Here's how the part is built. I have some questions about the finished solid (model axes, mm). Face numbers are marked on the shaded views. A direction names the side the tool comes from. Round coordinates to 2 decimals unless told otherwise and drop trailing zeros. Loops run counter-clockwise (first coordinate to the right, second up) from the corner with the lowest first, then second, coordinate; pieces in that order, holes last. Notation, with made-up numbers: M 87.25,23.25 L 96.25,23.25 A31 ccw 96.25,58.25 Z; hole C 67,23.5 d11. An arc over 180 degrees is marked long. Answer as a JSON object with one key per item and string values.
from build123d import *

# Parameters (mm, degrees)
BOSS_EXTRUDE1_DEPTH = 7.5
BOSS_EXTRUDE2_DEPTH = 7.5
DRAFT2_START        = -54.946043165
DRAFT2_DEPTH        = 100
DRAFT2_2_DEPTH      = 25
DRAFT2_START_2      = -29.946043165
DRAFT2_3_DEPTH      = 25
DRAFT2_START_3      = -4.946043165
DRAFT2_4_DEPTH      = 25
DRAFT2_START_4      = 20.053956835
DRAFT2_5_DEPTH      = 25
DRAFT2_START_5      = 35.053956835
DRAFT2_6_DEPTH      = 30
DRAFT2_START_6      = 65.053956835
DRAFT2_7_DEPTH      = 30
SKETCH3_W           = 64.747590887
SKETCH3_H           = 7.5
BOSS_EXTRUDE3_DEPTH = 7.5
CUT_EXTRUDE1_DEPTH  = 3.8
CUT_EXTRUDE2_DEPTH  = 3.8
LPATTERN1_COUNT     = 2
LPATTERN1_PITCH     = 25


# Read off the part's stored shape, not the designer's step: Draft2
with BuildPart() as part:
    # Sketch1 → Boss-Extrude1 (new body)
    with BuildSketch(Plane.XY):
        Polygon((-40.366906475, -54.946043165), (22.633093525, -54.946043165), (22.633093525, -29.946043165), (30.633093525, -29.946043165), (30.633093525, -4.946043165), (22.633093525, -4.946043165), (22.633093525, 20.053956835), (30.633093525, 20.053956835), (30.633093525, 45.053956835), (-32.366906475, 45.053956835), (-32.366906475, 20.053956835), (-40.366906475, 20.053956835), (-40.366906475, -4.946043165), (-32.366906475, -4.946043165), (-32.366906475, -29.946043165), (-40.366906475, -29.946043165), align=None)
    extrude(amount=BOSS_EXTRUDE1_DEPTH)

    # Sketch2 → Boss-Extrude2 (add)
    with BuildSketch(Plane.XY.offset(7.5)):
        Polygon((-48.166906475, 35.053956835), (30.633093525, 35.053956835), (30.633093525, 65.053956835), (38.633093525, 65.053956835), (38.633093525, 95.053956835), (-40.166906475, 95.053956835), (-40.166906475, 65.053956835), (-48.166906475, 65.053956835), align=None)
    extrude(amount=BOSS_EXTRUDE2_DEPTH)

    # Draft2 outline → Draft2 (add)
    with BuildSketch(Plane(origin=(0, 0, 0), x_dir=(1, 0, 0), z_dir=(0, 1, 0)).offset(DRAFT2_START)):
        Polygon((-32.366906475, 0), (-37.240701918, 0), (-34.803804197, -7.5), (-32.366906475, -7.5), align=None)
        Polygon((27.506888969, 0), (22.633093525, 0), (22.633093525, -7.5), (25.069991247, -7.5), align=None)
    extrude(amount=DRAFT2_DEPTH)

    # Draft2 2 outline → Draft2 2 (add)
    with BuildSketch(Plane(origin=(0, 0, 0), x_dir=(1, 0, 0), z_dir=(0, 1, 0)).offset(DRAFT2_START)):
        Polygon((-40.366906475, 0), (-45.240701918, 0), (-42.803804197, -7.5), (-40.366906475, -7.5), align=None)
    extrude(amount=DRAFT2_2_DEPTH)

    # Draft2 3 outline → Draft2 3 (add)
    with BuildSketch(Plane(origin=(0, 0, 0), x_dir=(1, 0, 0), z_dir=(0, 1, 0)).offset(DRAFT2_START_2)):
        Polygon((35.506888969, 0), (30.633093525, 0), (30.633093525, -7.5), (33.069991247, -7.5), align=None)
    extrude(amount=DRAFT2_3_DEPTH)

    # Draft2 4 outline → Draft2 4 (add)
    with BuildSketch(Plane(origin=(0, 0, 0), x_dir=(1, 0, 0), z_dir=(0, 1, 0)).offset(DRAFT2_START_3)):
        Polygon((-40.366906475, 0), (-45.240701918, 0), (-42.803804197, -7.5), (-40.366906475, -7.5), align=None)
    extrude(amount=DRAFT2_4_DEPTH)

    # Draft2 5 outline → Draft2 5 (add)
    with BuildSketch(Plane(origin=(0, 0, 0), x_dir=(1, 0, 0), z_dir=(0, 1, 0)).offset(DRAFT2_START_4)):
        Polygon((35.506888969, 0), (30.633093525, 0), (30.633093525, -7.5), (33.069991247, -7.5), align=None)
    extrude(amount=DRAFT2_5_DEPTH)

    # Draft2 6 outline → Draft2 6 (add)
    with BuildSketch(Plane(origin=(0, 0, 0), x_dir=(1, 0, 0), z_dir=(0, 1, 0)).offset(DRAFT2_START_5)):
        Polygon((-48.166906475, -15), (-48.166906475, -7.5), (-50.603804197, -7.5), align=None)
        Polygon((33.069991247, -7.5), (30.633093525, -7.5), (30.633093525, -15), align=None)
    extrude(amount=DRAFT2_6_DEPTH)

    # Draft2 7 outline → Draft2 7 (add)
    with BuildSketch(Plane(origin=(0, 0, 0), x_dir=(1, 0, 0), z_dir=(0, 1, 0)).offset(DRAFT2_START_6)):
        Polygon((41.069991247, -7.5), (38.633093525, -7.5), (38.633093525, -15), align=None)
        Polygon((-40.166906475, -7.5), (-42.603804197, -7.5), (-40.166906475, -15), align=None)
    extrude(amount=DRAFT2_7_DEPTH)

    # Sketch3 → Boss-Extrude3 (add)
    with BuildSketch(Plane(origin=(0, 0, 0), x_dir=(-1, 0, 0), z_dir=(0, 0, -1))):
        with Locations((4.866906474, -51.196043165)):
            Rectangle(SKETCH3_W, SKETCH3_H)
    boss_extrude3 = extrude(amount=BOSS_EXTRUDE3_DEPTH)

    # Sketch4 → Cut-Extrude1 (cut)
    with BuildSketch(Plane.XZ.offset(54.946043165)):
        Polygon((27.506888969, -7.5), (27.506888969, 0), (20.278859445, -2.348529157), (20.278859445, -7.5), align=None)
    cut_extrude1 = extrude(amount=-CUT_EXTRUDE1_DEPTH, mode=Mode.SUBTRACT)

    # Sketch5 → Cut-Extrude2 (cut)
    with BuildSketch(Plane(origin=(0, -47.446043165, 0), x_dir=(1, 0, 0), z_dir=(0, 1, 0))):
        Polygon((-37.240701918, 7.5), (-37.240701918, 0), (-30.012672394, 2.348529157), (-30.012672394, 7.5), align=None)
    cut_extrude2 = extrude(amount=-CUT_EXTRUDE2_DEPTH, mode=Mode.SUBTRACT)

    # LPattern1: Boss-Extrude3, Cut-Extrude1, Cut-Extrude2 ×2
    with Locations(*[(0, i * LPATTERN1_PITCH, 0) for i in range(1, LPATTERN1_COUNT)]):
        add(boss_extrude3)
        add(cut_extrude1, mode=Mode.SUBTRACT)
        add(cut_extrude2, mode=Mode.SUBTRACT)

    # Chamfer2
    # the kernel refuses this chamfer: 5 mm, written as the material it takes off along each edge
    with BuildSketch(Plane(origin=(-40.441261641, -51.612709832, 4.248239139), x_dir=(-0.7189342036162105, 0.6942471081166146, 0.033978872000742164), z_dir=(-0.4932114534551065, -0.5439749702030539, 0.6788473274406317))) as chamfer2_piece_1:
        Polygon((-3.286728939, 2.231187156), (3.915317626, 2.231187156), (-0.628588687, -4.462374312), align=None)
    extrude(amount=5.70452533, mode=Mode.SUBTRACT)
    with BuildSketch(Plane(origin=(33.069991247, -42.853897845, 7.5), x_dir=(-0.9997407638607628, 0, 0.022768510603425433), z_dir=(0, 1, 0))) as chamfer2_piece_2:
        with BuildLine():
            Line((5.163141872, 0), (-1.817393185, -4.83271311))
            Line((-1.817393185, -4.83271311), (-1.911770596, -4.799654007))
            ThreePointArc((-1.911770596, -4.799654007), (-0.947600353, -2.402729105), (-0.094377411, 0.033059103))
            Line((-0.094377411, 0.033059103), (0.002276851, 0.099974076))
            ThreePointArc((0.002276851, 0.099974076), (2.582509488, 0.041210789), (5.165418723, 0.099974076))
            Line((5.165418723, 0.099974076), (5.163141872, 0))
        make_face()
    extrude(amount=50.815709359, mode=Mode.SUBTRACT)
    with BuildSketch(Plane(origin=(-49.214170654, -54.946043165, -12.229079318), x_dir=(0.9506969379377622, -0.027495876610586285, -0.30890016018962835), z_dir=(0.309016994289291, 0, 0.951056516322985))) as chamfer2_piece_3:
        with BuildLine():
            Line((5.143365976, 0), (-0.282735774, 5.135588968))
            Line((-0.282735774, 5.135588968), (-0.382697966, 5.13283938))
            ThreePointArc((-0.382697966, 5.13283938), (-0.170646135, 2.566989148), (-0.099962192, -0.002749588))
            Line((-0.099962192, -0.002749588), (0.002749588, -0.099962192))
            ThreePointArc((0.002749588, -0.099962192), (2.572488324, -0.029278248), (5.146115564, -0.099962192))
            Line((5.146115564, -0.099962192), (5.143365976, 0))
        make_face()
    extrude(amount=33.602796561, mode=Mode.SUBTRACT)
    with BuildSketch(Plane(origin=(33.069991247, 7.146102155, 7.5), x_dir=(-0.9997407638607628, 0, 0.022768510603425433), z_dir=(0, 1, 0))) as chamfer2_piece_4:
        with BuildLine():
            Line((5.163141872, 0), (-1.817393185, -4.83271311))
            Line((-1.817393185, -4.83271311), (-1.911770596, -4.799654007))
            ThreePointArc((-1.911770596, -4.799654007), (-0.947600353, -2.402729105), (-0.094377411, 0.033059103))
            Line((-0.094377411, 0.033059103), (0.002276851, 0.099974076))
            ThreePointArc((0.002276851, 0.099974076), (2.582509488, 0.041210789), (5.165418723, 0.099974076))
            Line((5.165418723, 0.099974076), (5.163141872, 0))
        make_face()
    extrude(amount=27.90785468, mode=Mode.SUBTRACT)
    with BuildSketch(Plane(origin=(-42.803804197, -67.853897845, 7.5), x_dir=(0.9997407638607191, 0, 0.022768510605345404), z_dir=(0, 1, 0)), Plane(origin=(-42.803804197, -17.853897845, 7.5), x_dir=(0.9997407638607191, 0, 0.022768510605345404), z_dir=(0, 1, 0))) as chamfer2_piece_5:
        with BuildLine():
            Line((5.163141872, 0), (-1.817393184, 4.83271311))
            Line((-1.817393184, 4.83271311), (-1.911770595, 4.799654007))
            ThreePointArc((-1.911770595, 4.799654007), (-0.947600353, 2.402729105), (-0.094377411, -0.033059103))
            Line((-0.094377411, -0.033059103), (0.002276851, -0.099974076))
            ThreePointArc((0.002276851, -0.099974076), (2.582509488, -0.041210789), (5.165418723, -0.099974076))
            Line((5.165418723, -0.099974076), (5.163141872, 0))
        make_face()
    extrude(amount=50.815709359, mode=Mode.SUBTRACT)
    with BuildSketch(Plane(origin=(-48.166906475, 77.961811514, 15), x_dir=(0.9997407638607629, 0, 0.022768510603425628), z_dir=(0, -1, 0)), Plane(origin=(38.633093525, 52.146102155, 15), x_dir=(-0.9997407638607629, 0, 0.022768510603425628), z_dir=(0, 1, 0))) as chamfer2_piece_6:
        with BuildLine():
            Line((5.163141872, 0), (-1.817393185, -4.83271311))
            Line((-1.817393185, -4.83271311), (-1.911770596, -4.799654007))
            ThreePointArc((-1.911770596, -4.799654007), (-0.947600353, -2.402729105), (-0.094377411, 0.033059103))
            Line((-0.094377411, 0.033059103), (0.002276851, 0.099974076))
            ThreePointArc((0.002276851, 0.099974076), (2.582509488, 0.041210789), (5.165418723, 0.099974076))
            Line((5.165418723, 0.099974076), (5.163141872, 0))
        make_face()
    extrude(amount=55.815709359, mode=Mode.SUBTRACT)
    with BuildSketch(Plane(origin=(-32.366906475, -54.946043165, 7.5), x_dir=(0, -0.027495876610586317, -0.9996219169112968), z_dir=(1, 0, 0))) as chamfer2_piece_7:
        with BuildLine():
            Line((5.143365976, 0), (-0.282735774, 5.135588968))
            Line((-0.282735774, 5.135588968), (-0.382697966, 5.13283938))
            ThreePointArc((-0.382697966, 5.13283938), (-0.170646135, 2.566989148), (-0.099962192, -0.002749588))
            Line((-0.099962192, -0.002749588), (0.002749588, -0.099962192))
            ThreePointArc((0.002749588, -0.099962192), (2.572488324, -0.029278248), (5.146115564, -0.099962192))
            Line((5.146115564, -0.099962192), (5.143365976, 0))
        make_face()
    extrude(amount=55, mode=Mode.SUBTRACT)
    with BuildSketch(Plane(origin=(-34.803804197, -54.946043165, 7.5), x_dir=(0, -0.02749587670275982, -0.9996219169087613), z_dir=(1, 0, 0))) as chamfer2_piece_8:
        with BuildLine():
            Line((5.143365976, 0), (-0.282735775, 5.135588968))
            Line((-0.282735775, 5.135588968), (-0.382697967, 5.13283938))
            ThreePointArc((-0.382697967, 5.13283938), (-0.170646136, 2.566989148), (-0.099962192, -0.002749588))
            Line((-0.099962192, -0.002749588), (0.002749588, -0.099962192))
            ThreePointArc((0.002749588, -0.099962192), (2.572488324, -0.029278248), (5.146115564, -0.099962192))
            Line((5.146115564, -0.099962192), (5.143365976, 0))
        make_face()
    extrude(amount=2.436897722, mode=Mode.SUBTRACT)
    with BuildSketch(Plane(origin=(22.633093525, -54.946043165, 7.5), x_dir=(0, -0.02749587670275982, -0.9996219169087613), z_dir=(1, 0, 0))) as chamfer2_piece_9:
        with BuildLine():
            Line((5.143365976, 0), (-0.282735775, 5.135588968))
            Line((-0.282735775, 5.135588968), (-0.382697967, 5.13283938))
            ThreePointArc((-0.382697967, 5.13283938), (-0.170646136, 2.566989148), (-0.099962192, -0.002749588))
            Line((-0.099962192, -0.002749588), (0.002749588, -0.099962192))
            ThreePointArc((0.002749588, -0.099962192), (2.572488324, -0.029278248), (5.146115564, -0.099962192))
            Line((5.146115564, -0.099962192), (5.143365976, 0))
        make_face()
    extrude(amount=15.295312662, mode=Mode.SUBTRACT)
    with BuildSketch(Plane(origin=(-40.366906475, -54.946043165, 7.5), x_dir=(0, -0.027495876610586317, -0.9996219169112968), z_dir=(1, 0, 0))) as chamfer2_piece_10:
        with BuildLine():
            Line((5.143365976, 0), (-0.282735774, 5.135588968))
            Line((-0.282735774, 5.135588968), (-0.382697966, 5.13283938))
            ThreePointArc((-0.382697966, 5.13283938), (-0.170646135, 2.566989148), (-0.099962192, -0.002749588))
            Line((-0.099962192, -0.002749588), (0.002749588, -0.099962192))
            ThreePointArc((0.002749588, -0.099962192), (2.572488324, -0.029278248), (5.146115564, -0.099962192))
            Line((5.146115564, -0.099962192), (5.143365976, 0))
        make_face()
    extrude(amount=5.563102278, mode=Mode.SUBTRACT)
    with BuildSketch(Plane(origin=(-55.662219137, -54.946043165, 7.5), x_dir=(0, -0.027495876610586317, -0.9996219169112968), z_dir=(1, 0, 0))) as chamfer2_piece_11:
        with BuildLine():
            Line((5.143365976, 0), (-0.282735774, 5.135588968))
            Line((-0.282735774, 5.135588968), (-0.382697966, 5.13283938))
            ThreePointArc((-0.382697966, 5.13283938), (-0.170646135, 2.566989148), (-0.099962192, -0.002749588))
            Line((-0.099962192, -0.002749588), (0.002749588, -0.099962192))
            ThreePointArc((0.002749588, -0.099962192), (2.572488324, -0.029278248), (5.146115564, -0.099962192))
            Line((5.146115564, -0.099962192), (5.143365976, 0))
        make_face()
    extrude(amount=15.295312662, mode=Mode.SUBTRACT)


solid = part.part
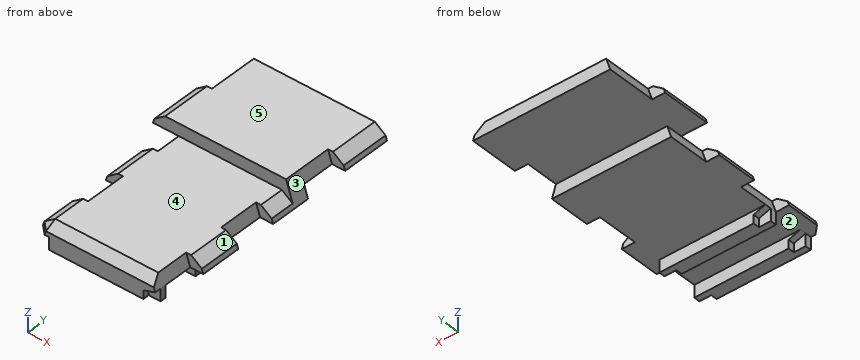
Item 1: I want a section at B-B, the plane y = 38.5. Please give me the cut outline in (x, z), then the cut area to 3 significant figures.
Resolved:
{"outline": "M -50.6,7.5 L -34.8,7.5 L -37.24,0 L 35.51,0 L 30.63,15 L -43.17,15 L -49.71,10.24 Z", "area": "1,120 mm²"}
Item 2: I want a section at A-A, the plane x = -5. Please give me the cut outline in (y, z).
Resolved:
{"outline": "M -54.95,-7.5 L -47.45,-7.5 L -47.45,0 L -29.95,0 L -29.95,-7.5 L -22.45,-7.5 L -22.45,0 L 45.05,0 L 45.05,7.5 L 95.05,7.5 L 95.05,15 L 35.05,15 L 35.05,7.5 L -49.95,7.5 L -54.95,2.5 Z"}
Item 3: I'm going to push flat-ended pins straight in: pin 1 Ø3.5 at (x, z) = (25, -3.5) entering from -Y; pin 2 Ø2 at (x, z) = (36, 12.5) entering from -Y; pin 3 Ø12 at (x, y) = (26, 65) entering from -Z; pin 4 Ø1 at (y, z) = (-2.5, -1.5) entering from -X. Where does each tip first touch, or does it pass through?
Resolved:
{"pin 1": "y = -51.15", "pin 2": "y = 65.05", "pin 3": "z = 7.5", "pin 4": "through"}
Item 4: I want a section at D-D, the plane y = 54.5. Please give me the cut outline in (x, z), then the cut area to 3 significant figures.
Resolved:
{"outline": "M -50.6,7.5 L 33.07,7.5 L 30.63,15 L -43.17,15 L -49.71,10.24 Z", "area": "597 mm²"}
Item 5: On a 3-axis mill with a long thin cutter (end or side, diameter ignored), from which of +Z, -Z, +X, -X, +Y, -Y can I reach the whole of each face in a straight line? I mean the marked faces 3, 4 and 5. Say none if no direction works.
Resolved:
{"face 3": "+Z, +X, -Y", "face 4": "+Z, +X, -X, -Y", "face 5": "+Z, +X, -X, +Y, -Y"}
Item 6: If we mould it in two halves opening along Y, with no side actions, what happens to the marked faces 1 and 2? For each: pulls with the +Y half, pulls with the -Y half, needs draft (parallel to the pull), parting line crosses it, or undercut.
Resolved:
{"face 1": "needs draft", "face 2": "undercut"}
Item 7: Please list where these lines run through material, in increasing order: probe 1 along Y at (x, z) = (-6, -1); probe 2 along Z at (x, y) = (20, -21); probe 3 along Y at (x, z) = (-2, 14.25). Write a range as from..to.
Resolved:
{"probe 1": "-54.95..-47.45, -29.95..-22.45", "probe 2": "0..7.5", "probe 3": "35.05..95.05"}
Item 8: I want a section at C-C, the plane z = 5.75. Please give me the cut outline in (x, y).
Resolved:
{"outline": "M -40.21,-49.95 L -38.28,-51.7 L 25.64,-51.7 L 25.64,-29.95 L 30.48,-29.95 L 30.48,-4.95 L 25.64,-4.95 L 25.64,20.05 L 30.48,20.05 L 30.48,35.05 L 33.64,35.05 L 33.64,45.05 L -35.37,45.05 L -35.37,20.05 L -40.21,20.05 L -40.21,-4.95 L -35.37,-4.95 L -35.37,-29.95 L -40.21,-29.95 Z"}
